CAD build for the part. Positions are in the model's coordinates, mm. Round coordinates to 2 decimals unless told otherwise and drop trailing zeros. Write each loop counter-clockwise with the first axis right and the second up, starting at its lowest first coordinate (ties: lowest second). Pieces come first, ordered by that corner, then holes. Notation, with made-up numbers: (38.25, -31) -> (45.25, -31) arc R24 ccw to (45.25, -17) -> close; hole circle Ø6 at (86, 47). An arc over 180 degrees is marked (long way). Put each result on its own line as item: value. Start each with the question number.
1. Saw through at A-A on z = 0. List the corners of the cut face in (x, y) (3 decimals).
2. Saw through at B-B on x = -117. List the corners of the cut face in (y, z) (3 decimals), and give its area (3 significant figures).
3. Drill centre lines: line 1 (X direction, y = -1, z = 0.5); line 2 (Z direction, x = 117, y = -0.75); line 3 (X direction, y = -2.5, z = 1.25). Where is each one in solid material? Low to high. Write a range as from..to.
4. Flat gauge pins, fed straight in: P1, Ø7, axis at x = -117, z = 0, coming from the -Y side (3 decimals); P2, Ø1.5, axis at y = -1, z = -9.5, coming from the -X side. Where does each tip first touch, or does it go through?
5. Pull direction Z, two halves, no side cores. Call faces 1 (the flat face through (-2, -3.175, 0)), 2 (the cylindrical face through (-128.5, -1.57, 11.07)), 3 (the cylindrical face through (-114.043, -1.565, 0.931)): pulls with the +Z half, pulls with the -Z half, needs draft (parallel to the pull), parting line crosses it, or undercut.
from build123d import *

# Parameters (mm, degrees)
F0_R     = 3.1
F1_DEPTH = 3.175


with BuildPart() as f1:
    # F0 (on Front) → F1 (new body)
    with BuildSketch(Plane.XZ):
        with BuildLine():
            Line((125, 12.5), (-125, 12.5))
            ThreePointArc((-125, 12.5), (-128.535534, 11.035534), (-130, 7.5))
            Line((-130, 7.5), (-130, -7.5))
            ThreePointArc((-130, -7.5), (-128.535534, -11.035534), (-125, -12.5))
            Line((-125, -12.5), (125, -12.5))
            ThreePointArc((125, -12.5), (128.535534, -11.035534), (130, -7.5))
            Line((130, -7.5), (130, 7.5))
            ThreePointArc((130, 7.5), (128.535534, 11.035534), (125, 12.5))
        make_face()
        with Locations((-117, 0)):
            Circle(F0_R, mode=Mode.SUBTRACT)
        with BuildLine():
            ThreePointArc((120.1, 0), (117, -3.1), (113.9, 0))
            ThreePointArc((113.9, 0), (117, 3.1), (120.1, 0))
        make_face(mode=Mode.SUBTRACT)
    extrude(amount=F1_DEPTH)


solid = f1.part
Return value:
1. outline: (-130, -3.175) -> (-120.1, -3.175) -> (-120.1, 0) -> (-130, 0) -> close; (-113.9, -3.175) -> (113.9, -3.175) -> (113.9, 0) -> (-113.9, 0) -> close; (120.1, -3.175) -> (130, -3.175) -> (130, 0) -> (120.1, 0) -> close
2. outline: (-3.175, -12.5) -> (0, -12.5) -> (0, -3.1) -> (-3.175, -3.1) -> close; (-3.175, 3.1) -> (0, 3.1) -> (0, 12.5) -> (-3.175, 12.5) -> close
2. area: 59.7 mm^2
3. line 1: x = -130..-120.06, -113.94..113.94, 120.06..130
3. line 2: z = -12.5..-3.1, 3.1..12.5
3. line 3: x = -130..-119.84, -114.16..114.16, 119.84..130
4. P1: stops at y = -3.175
4. P2: stops at x = -129.84
5. face 1: needs draft
5. face 2: pulls with the +Z half
5. face 3: undercut
